Build history of the part. All positions in model axes, mm. A direction names the side the tool comes from. Give positions to 0.01 mm unless a question says otherwise; leave off trailing zeros. Write each loop counter-clockwise with the first axis right and the second up, starting at its lowest first coordinate (ties: lowest second). Pieces come first, ordered by that corner, then holes. Notation, with made-up numbers: (86.5, -11) -> (116.5, -11) arc R22 cw to (116.5, 8) -> close; hole circle Ø4 at (-18.75, 31.5). An arc over 180 degrees is marked (long way). Put each result on its own line as item: value.
from build123d import *

# Parameters (mm, degrees)
Y_KSEKLIK_EKSTR_ZYON1_DEPTH = 12
IZIM2_W                     = 50
IZIM2_H                     = 56
Y_KSEKLIK_EKSTR_ZYON2_DEPTH = 4
IZIM3_W                     = 38
IZIM3_H                     = 4
KES_EKSTR_ZYON1_DEPTH       = 56
IZIM4_R                     = 5
KES_EKSTR_ZYON2_DEPTH       = 56
KES_EKSTR_ZYON3_DEPTH       = 56


with BuildPart() as part:
    # Çizim1 → Yükseklik-Ekstrüzyon1 (new body)
    with BuildSketch(Plane(origin=(0, 0, 0), x_dir=(1, 0, 0), z_dir=(0, 1, 0))):
        Polygon((69.99751861, 24.903225806), (69.99751861, -31.096774194), (-58.00248139, -31.096774194), (-58.00248139, 24.903225806), (-19.00248139, 24.903225806), (30.99751861, 24.903225806), align=None)
    extrude(amount=Y_KSEKLIK_EKSTR_ZYON1_DEPTH)

    # Çizim2 → Yükseklik-Ekstrüzyon2 (add)
    with BuildSketch(Plane(origin=(0, 12, 0), x_dir=(1, 0, 0), z_dir=(0, 1, 0))):
        with Locations((5.99751861, -3.096774194)):
            Rectangle(IZIM2_W, IZIM2_H)
    extrude(amount=Y_KSEKLIK_EKSTR_ZYON2_DEPTH)

    # Çizim3 → Kes-Ekstrüzyon1 (cut)
    with BuildSketch(Plane.XY.offset(31.096774194)):
        with Locations((5.99751861, 2)):
            Rectangle(IZIM3_W, IZIM3_H)
    extrude(amount=-KES_EKSTR_ZYON1_DEPTH, mode=Mode.SUBTRACT)

    # Çizim4 → Kes-Ekstrüzyon2 (cut)
    with BuildSketch(Plane(origin=(0, 12, 0), x_dir=(1, 0, 0), z_dir=(0, 1, 0))):
        with Locations((-48.00248139, 11.903225806)):
            Circle(IZIM4_R)
        with Locations((-48.00248139, -18.096774194)):
            Circle(IZIM4_R)
        with Locations((59.99751861, -18.096774194)):
            Circle(IZIM4_R)
        with Locations((59.99751861, 11.903225806)):
            Circle(IZIM4_R)
    extrude(amount=-KES_EKSTR_ZYON2_DEPTH, mode=Mode.SUBTRACT)

    # Çizim5 → Kes-Ekstrüzyon3 (cut)
    with BuildSketch(Plane(origin=(0, 12, 0), x_dir=(1, 0, 0), z_dir=(0, 1, 0))):
        with BuildLine():
            Line((-58.00248139, 19.903225806), (-58.00248139, 24.903225806))
            Line((-58.00248139, 24.903225806), (-53.00248139, 24.903225806))
            ThreePointArc((-53.00248139, 24.903225806), (-56.538015296, 23.438759712), (-58.00248139, 19.903225806))
        make_face()
        with BuildLine():
            Line((69.99751861, -26.096774194), (69.99751861, -31.096774194))
            Line((69.99751861, -31.096774194), (64.99751861, -31.096774194))
            ThreePointArc((64.99751861, -31.096774194), (68.533052516, -29.632308099), (69.99751861, -26.096774194))
        make_face()
        with BuildLine():
            Line((-58.00248139, -31.096774194), (-53.00248139, -31.096774194))
            ThreePointArc((-53.00248139, -31.096774194), (-56.538015296, -29.632308099), (-58.00248139, -26.096774194))
            Line((-58.00248139, -26.096774194), (-58.00248139, -31.096774194))
        make_face()
        with BuildLine():
            Line((69.99751861, 24.903225806), (64.99751861, 24.903225806))
            ThreePointArc((64.99751861, 24.903225806), (68.533052516, 23.438759712), (69.99751861, 19.903225806))
            Line((69.99751861, 19.903225806), (69.99751861, 24.903225806))
        make_face()
    extrude(amount=-KES_EKSTR_ZYON3_DEPTH, mode=Mode.SUBTRACT)


solid = part.part
1) Slice it at B-B (z = -15.5). Write the cut outline in (x, y), plus the area to 3 significant figures.
Filled sheet:
outline: (-58, 0) -> (-51.48, 0) -> (-51.48, 12) -> (-58, 12) -> close; (-44.53, 0) -> (-13, 0) -> (-13, 4) -> (25, 4) -> (25, 0) -> (56.52, 0) -> (56.52, 12) -> (31, 12) -> (31, 16) -> (-19, 16) -> (-19, 12) -> (-44.53, 12) -> close; (63.47, 0) -> (70, 0) -> (70, 12) -> (63.47, 12) -> close
area: 1,420 mm2
2) Pin check, flat tips, straight feed: pin 1 (13 mm diameter, centred on x = 60, z = -11.9, fed in from +Y); pin 2 (11.5 mm diameter, centred on x = -2, z = 13, fed in from -Y); pin 3 (4.5 mm diameter, centred on y = 15, z = -1, fed in from +X); pin 4 (11.5 mm diameter, centred on x = -48, z = 18.1, fed in from -Y). Stop position of each tip, or through.
Filled sheet:
pin 1: y = 12
pin 2: y = 4
pin 3: x = 31
pin 4: y = 0
3) Wall check: L1, parallel to Z at x = -48.5, y = 1; L2, parallel to X at y = 2.75, z = -8.5; L3, parallel to X at y = 8, z = 21.5. Give the ranges that are in metal, low to high.
Filled sheet:
L1: -24.9 to -16.88, -6.93 to 13.12, 23.07 to 31.1
L2: -58 to -51.67, -44.34 to -13, 25 to 56.33, 63.66 to 70
L3: -58 to -51.67, -44.34 to 56.33, 63.66 to 70
4) Slice it at C-C (y = 9.75). Write the cut outline in (x, z), plus the area to 3 significant figures.
Filled sheet:
outline: (-58, -19.9) arc R5 ccw to (-53, -24.9) -> (65, -24.9) arc R5 ccw to (70, -19.9) -> (70, 26.1) arc R5 ccw to (65, 31.1) -> (-53, 31.1) arc R5 ccw to (-58, 26.1) -> close; hole circle Ø10 at (-48, -11.9); hole circle Ø10 at (-48, 18.1); hole circle Ø10 at (60, -11.9); hole circle Ø10 at (60, 18.1)
area: 6,830 mm2
5) Slice it at D-D (z = 7). Write the cut outline in (x, y).
Filled sheet:
outline: (-58, 0) -> (-13, 0) -> (-13, 4) -> (25, 4) -> (25, 0) -> (70, 0) -> (70, 12) -> (31, 12) -> (31, 16) -> (-19, 16) -> (-19, 12) -> (-58, 12) -> close
6) Tool access for faces 4 (the flat face through (24.998, 2, 3)), 5 (the flat face through (-38, 12, 3)), 6 (the flat face through (51, 12, 3)): list every direction of +Z, -Z, +X, -X, +Y, -Y with a clear straight run to the whole face (end or side of a thin tool).
Filled sheet:
face 4: +Z, -Z, -Y
face 5: +Z, -Z, -X, +Y
face 6: +Z, -Z, +X, +Y
7) Slice it at A-A (x = 60). Write the cut outline in (y, z), plus the area to 3 significant figures.
Filled sheet:
outline: (0, -24.9) -> (12, -24.9) -> (12, -16.9) -> (0, -16.9) -> close; (0, -6.9) -> (12, -6.9) -> (12, 13.1) -> (0, 13.1) -> close; (0, 23.1) -> (12, 23.1) -> (12, 31.1) -> (0, 31.1) -> close
area: 432 mm2
8) Pull direction X, two halves, no side cores. Call faces 1 (the flat face through (7, 8, 31.097)), 2 (the flat face through (-19.002, 14, 3)), 3 (the cylindrical face through (56.31, 6.08, -15.28)): released by +X, released by -X, zero draft, split by the parting line, or undercut.
Filled sheet:
face 1: zero draft
face 2: released by -X
face 3: undercut
